The listing builds one solid part. Answer for the finished solid, in the listing's coordinates (mm). A direction names the side the tool comes from. Coordinates: 2 decimals unless noted, no trailing zeros. Order: outer loops, then holes, each group sorted by start corner. A loop starts at its lowest first (then second) coordinate and runs counter-clockwise, first axis right, second up. Notation, with made-up numbers: (40.25, 18.25) - (88.25, 18.25) arc R13 cw to (88.25, 39.25) - close; hole circle Ø11 at (42.25, 37). An arc over 180 degrees is marked (long way). Use a Markdown table: item, result. Add a question column.
Item 1: The part is cut by section C-C, the plane x = 258.5. Give the vertices of the cut face in (y, z), then the cut area to 3 significant figures.
Item 2: Find the intervals of material crossed by line 1 along Z through (x, y) = (312, 75); line 2 along Y through (x, z) = (197, -1306); line 3 along Z through (x, y) = (70, -189), in increasing order.
Item 3: The part is cut by section A-A, the plane z = -544. Give the vertices of the cut face in (x, y).
Item 4: The mould has two halves that part along Z. Classify faces 4 (the flat face through (-421.5, -144, -2096)), 5 (the flat face through (-451.08, -143.88, -130.28)), 6 (the flat face through (-446, -151, -2180)), 7 (the flat face through (501.5, 145, -9)): released by +Z, released by -Z, zero draft, split by the parting line, or undercut.
Item 5: Flat-ended cylindrical pins translate along their axes: P1, Ø1.5, axis at x = 113.5, z = -1530, coming from the -Y side; P2, Ø5, axis at x = 159, z = -1476.5, coming from the +Y side; P3, Ø21, axis at x = -431, y = -176, coming from the +Z side. Find the tip coordinate at first contact, or state that the pin passes through.
Item 6: The part is cut by section B-B, the plane y = 140. Give the vertices of the cut face in (x, z), then the cut area to 3 significant figures.
Item 7: The part is cut by section D-D, the plane y = -114.5. State how many separate pieces and enclosed holes the cut face has, then the cut area to 3 significant figures.
Item 8: For faces 1 (the flat face through (446, -154, -2180)), 2 (the flat face through (421.5, -144, -2096)), 3 (the flat face through (451.08, -143.88, -2049.72)), determine the directions among +Z, -Z, +X, -X, +Y, -Y from which every point of the face is accessible in a straight line to the end or side of a thin tool.
from build123d import *

# Parameters (mm, degrees)
SKETCH1_W                = 40
SKETCH1_H                = 40
SKETCH1_H_2              = 10
SKETCH1_W_2              = 903
SKETCH1_H_3              = 2060
BOSS_EXTRUDE1_DEPTH      = 65
BOSS_EXTRUDE2_DEPTH      = 350
BOSS_EXTRUDE2_DEPTH_BACK = 50
SKETCH1_3_W              = 943
SKETCH1_3_H              = 80
SKETCH1_3_H_2            = 101
SKETCH1_4_W              = 40
SKETCH1_4_H              = 40
BOSS_EXTRUDE3_DEPTH      = 240
BOSS_EXTRUDE4_DEPTH      = 30
BOSS_EXTRUDE5_DEPTH      = 30
SKETCH5_W                = 30
SKETCH5_H                = 30
CUT_EXTRUDE1_DEPTH       = 200
BOSS_EXTRUDE6_DEPTH      = 30
BOSS_EXTRUDE7_START      = -30
BOSS_EXTRUDE7_DEPTH      = 30
BOSS_EXTRUDE8_DEPTH      = 20
BOSS_EXTRUDE8_DEPTH_BACK = 20
SKETCH8_W                = 743
SKETCH8_H                = 450
BOSS_EXTRUDE9_DEPTH      = 130
BOSS_EXTRUDE14_DEPTH     = 30
BOSS_EXTRUDE15_DEPTH     = 30
BOSS_EXTRUDE16_DEPTH     = 30
BOSS_EXTRUDE17_DEPTH     = 30
BOSS_EXTRUDE18_DEPTH     = 30
BOSS_EXTRUDE19_DEPTH     = 30


with BuildPart() as part:
    # Sketch1 → Boss-Extrude1 (new body)
    with BuildSketch(Plane(origin=(0, 0, 0), x_dir=(1, 0, 0), z_dir=(0, 1, 0))):
        with Locations((-431.5, 20)):
            Rectangle(SKETCH1_W, SKETCH1_H)
        Polygon((-411.5, 50), (-411.5, 40), (-411.5, 0), (411.5, 0), (411.5, 40), (411.5, 50), align=None)
        with Locations((-431.5, 45)):
            Rectangle(SKETCH1_W, SKETCH1_H_2)
        Polygon((-451.5, 0), (-451.5, 40), (-451.5, 50), (-451.5, 60), (-471.5, 60), (-471.5, -41), (471.5, -41), (471.5, 60), (451.5, 60), (451.5, 50), (451.5, 40), (451.5, 0), (411.5, 0), (-411.5, 0), align=None)
        Polygon((-451.5, 50), (-411.5, 50), (411.5, 50), (451.5, 50), (451.5, 60), (-451.5, 60), align=None)
        with Locations((431.5, 20)):
            Rectangle(SKETCH1_W, SKETCH1_H)
        with Locations((431.5, 45)):
            Rectangle(SKETCH1_W, SKETCH1_H_2)
        with Locations((0, 1090)):
            Rectangle(SKETCH1_W_2, SKETCH1_H_3)
        Polygon((-471.5, 2120), (-451.5, 2120), (-451.5, 2130), (-451.5, 2140), (-451.5, 2180), (-411.5, 2180), (411.5, 2180), (451.5, 2180), (451.5, 2140), (451.5, 2130), (451.5, 2120), (471.5, 2120), (471.5, 2200), (-471.5, 2200), align=None)
        Polygon((-451.5, 2130), (-451.5, 2120), (451.5, 2120), (451.5, 2130), (411.5, 2130), (-411.5, 2130), align=None)
        with Locations((-431.5, 2135)):
            Rectangle(SKETCH1_W, SKETCH1_H_2)
        with Locations((-431.5, 2160)):
            Rectangle(SKETCH1_W, SKETCH1_H)
        Polygon((-411.5, 2140), (-411.5, 2130), (411.5, 2130), (411.5, 2140), (411.5, 2180), (-411.5, 2180), align=None)
        with Locations((431.5, 2135)):
            Rectangle(SKETCH1_W, SKETCH1_H_2)
        with Locations((431.5, 2160)):
            Rectangle(SKETCH1_W, SKETCH1_H)
    extrude(amount=-BOSS_EXTRUDE1_DEPTH)

    # Sketch1_3 → Boss-Extrude2 (add, two sides: drawn at the far end of the back side and taken through both)
    with BuildSketch(Plane(origin=(0, 0, 0), x_dir=(1, 0, 0), z_dir=(0, 1, 0)).offset(-BOSS_EXTRUDE2_DEPTH_BACK)):
        with Locations((0, 2160)):
            Rectangle(SKETCH1_3_W, SKETCH1_3_H)
        with Locations((0, 9.5)):
            Rectangle(SKETCH1_3_W, SKETCH1_3_H_2)
    extrude(amount=BOSS_EXTRUDE2_DEPTH + BOSS_EXTRUDE2_DEPTH_BACK)

    # Sketch1_4 → Boss-Extrude3 (add)
    with BuildSketch(Plane(origin=(0, 0, 0), x_dir=(1, 0, 0), z_dir=(0, 1, 0))):
        with Locations((431.5, 2160)):
            Rectangle(SKETCH1_4_W, SKETCH1_4_H)
        with Locations((-431.5, 2160)):
            Rectangle(SKETCH1_4_W, SKETCH1_4_H)
        with Locations((-431.5, 20)):
            Rectangle(SKETCH1_4_W, SKETCH1_4_H)
        with Locations((431.5, 20)):
            Rectangle(SKETCH1_4_W, SKETCH1_4_H)
    extrude(amount=-BOSS_EXTRUDE3_DEPTH)

    # Sketch3 → Boss-Extrude4 (add)
    with BuildSketch(Plane(origin=(451.5, 0, 0), x_dir=(0, 0, -1), z_dir=(1, 0, 0))):
        Polygon((40, -65), (40, -225), (110, -225), (150, -65), align=None)
        Polygon((2140, -65), (2030, -65), (2070, -225), (2140, -225), align=None)
    extrude(amount=-BOSS_EXTRUDE4_DEPTH)

    # Sketch4 → Boss-Extrude5 (add)
    with BuildSketch(Plane(origin=(-451.5, 0, -45.75), x_dir=(0, 0, -1), z_dir=(1, 0, 0))):
        Polygon((2024.25, -225), (2094.25, -225), (2094.25, -65), (1984.25, -65), align=None)
        Polygon((64.25, -225), (104.25, -65), (-5.75, -65), (-5.75, -225), align=None)
    extrude(amount=BOSS_EXTRUDE5_DEPTH)

    # Sketch5 → Cut-Extrude1 (cut)
    with BuildSketch(Plane.XZ.offset(240)):
        with Locations((-431.5, -2160)):
            Rectangle(SKETCH5_W, SKETCH5_H)
        with Locations((431.5, -2160)):
            Rectangle(SKETCH5_W, SKETCH5_H)
        with Locations((431.5, -20)):
            Rectangle(SKETCH5_W, SKETCH5_H)
        with Locations((-431.5, -20)):
            Rectangle(SKETCH5_W, SKETCH5_H)
    extrude(amount=-CUT_EXTRUDE1_DEPTH, mode=Mode.SUBTRACT)

    # Sketch6 → Boss-Extrude6 (add)
    with BuildSketch(Plane.XY.offset(41)):
        with BuildLine():
            Line((130, -65), (-130, -65))
            ThreePointArc((-130, -65), (0, -195), (130, -65))
        make_face()
    extrude(amount=-BOSS_EXTRUDE6_DEPTH)

    # Sketch7 → Boss-Extrude7 (add)
    with BuildSketch(Plane(origin=(0, 0, -2200), x_dir=(-1, 0, 0), z_dir=(0, 0, -1)).offset(BOSS_EXTRUDE7_START)):
        with BuildLine():
            Line((130, -65), (-130, -65))
            ThreePointArc((-130, -65), (0, -195), (130, -65))
        make_face()
    extrude(amount=BOSS_EXTRUDE7_DEPTH)

    # 3DSketch1 → Boss-Extrude8 (add, two sides: drawn at the far end of the back side and taken through both)
    with BuildSketch(Plane(origin=(0, -195, 11), x_dir=(0, 0.018337127203073178, -0.9998318607475651), z_dir=(1, 0, 0)).offset(-BOSS_EXTRUDE8_DEPTH_BACK)):
        Polygon((0, 0), (0.733485088, 39.99327443), (2181.366773379, 0), (2180.63328829, -39.99327443), align=None)
    extrude(amount=BOSS_EXTRUDE8_DEPTH + BOSS_EXTRUDE8_DEPTH_BACK)

    # Sketch8 → Boss-Extrude9 (add)
    with BuildSketch(Plane.XZ.offset(65)):
        with Locations((0, -184)):
            Rectangle(SKETCH8_W, SKETCH8_H)
    extrude(amount=BOSS_EXTRUDE9_DEPTH)

    # Sketch12 → Boss-Extrude14 (add)
    with BuildSketch(Plane.ZY.offset(451.5)):
        Polygon((-60, 0), (-2120, 0), (-2120, -65), (-2180, -65), (-2180, -240), (-2140, -240), (-2140, -225), (-2070, -225), (-2030, -65), (-150, -65), (-110, -225), (-40, -225), (-40, -240), (0, -240), (0, -65), (-60, -65), align=None)
    extrude(amount=BOSS_EXTRUDE14_DEPTH)

    # Sketch13 → Boss-Extrude15 (add)
    with BuildSketch(Plane(origin=(451.5, 0, 0), x_dir=(0, 0, -1), z_dir=(1, 0, 0))):
        Polygon((2120, 0), (60, 0), (60, -65), (0, -65), (0, -240), (40, -240), (40, -225), (110, -225), (150, -65), (2030, -65), (2070, -225), (2140, -225), (2140, -240), (2180, -240), (2180, -65), (2120, -65), align=None)
    extrude(amount=BOSS_EXTRUDE15_DEPTH)

    # Sketch14 → Boss-Extrude16 (add)
    with BuildSketch(Plane.ZY.offset(471.5)):
        Polygon((-2120, 350), (-2200, 350), (-2200, -65), (-2180, -65), (-2120, -65), (-2120, 0), align=None)
    extrude(amount=BOSS_EXTRUDE16_DEPTH)

    # Sketch15 → Boss-Extrude17 (add)
    with BuildSketch(Plane.ZY.offset(471.5)):
        Polygon((41, -65), (41, 350), (-60, 350), (-60, 0), (-60, -65), (0, -65), align=None)
    extrude(amount=BOSS_EXTRUDE17_DEPTH)

    # Sketch16 → Boss-Extrude18 (add)
    with BuildSketch(Plane(origin=(471.5, 0, 0), x_dir=(0, 0, -1), z_dir=(1, 0, 0))):
        Polygon((2200, 350), (2120, 350), (2120, 0), (2120, -65), (2180, -65), (2200, -65), align=None)
    extrude(amount=BOSS_EXTRUDE18_DEPTH)

    # Sketch17 → Boss-Extrude19 (add)
    with BuildSketch(Plane(origin=(471.5, 0, 0), x_dir=(0, 0, -1), z_dir=(1, 0, 0))):
        Polygon((60, -65), (60, 0), (60, 350), (-41, 350), (-41, -65), (0, -65), align=None)
    extrude(amount=BOSS_EXTRUDE19_DEPTH)


solid = part.part
Solution:
| question | item | result |
|---|---|---|
| 1 | outline | (-195, -409) - (-65, -409) - (-65, -2200) - (350, -2200) - (350, -2120) - (0, -2120) - (0, -60) - (350, -60) - (350, 41) - (-195, 41) - close |
| 1 | area | 268,000 mm2 |
| 2 | line 1 | z = -2200 to -2120, -60 to 41 |
| 2 | line 2 | y = -65 to 0 |
| 2 | line 3 | z = -409 to 41 |
| 3 | outline | (-481.5, -65) - (481.5, -65) - (481.5, 0) - (-481.5, 0) - close; (-20, -195) - (20, -195) - (20, -155) - (-20, -155) - close |
| 4 | face 4 | undercut |
| 4 | face 5 | undercut |
| 4 | face 6 | released by -Z |
| 4 | face 7 | zero draft |
| 5 | P1 | stops at y = -65 |
| 5 | P2 | stops at y = 0 |
| 5 | P3 | stops at z = 0 |
| 6 | outline | (-501.5, -2200) - (501.5, -2200) - (501.5, -2120) - (-501.5, -2120) - close; (-501.5, -60) - (501.5, -60) - (501.5, 41) - (-501.5, 41) - close |
| 6 | area | 182,000 mm2 |
| 7 | separate pieces | 6 |
| 7 | enclosed holes | 4 |
| 7 | area | 373,000 mm2 |
| 8 | face 1 | -Z, +X, -Y |
| 8 | face 2 | -Y |
| 8 | face 3 | +X, -Y |
